```python
from build123d import *

# Parameters (mm, degrees)
ESTRUSIONE_ESTRUSIONE1_DEPTH                 = 5
FORO_LAMATO_PER_VITE_M4_A_TESTA_CILI_2_COUNT = 2
FORO_LAMATO_PER_VITE_M4_A_TESTA_CILI_2_PITCH = 164
FORO_LAMATO_PER_VITE_M4_A_TESTA_CILI_3_COUNT = 2
FORO_LAMATO_PER_VITE_M4_A_TESTA_CILI_3_PITCH = 159
SCHIZZO5_R                                   = 1.75
SCHIZZO5_R_2                                 = 10
SCHIZZO5_R_3                                 = 11
SCHIZZO5_R_4                                 = 13
SCHIZZO5_R_5                                 = 4
SCHIZZO5_R_6                                 = 26
SCHIZZO5_W                                   = 39
SCHIZZO5_H                                   = 24
TAGLIO_ESTRUSIONE2_DEPTH                     = 7


with BuildPart() as part:
    # Schizzo1 → Estrusione-Estrusione1 (new body)
    with BuildSketch(Plane.XY):
        with BuildLine():
            Line((0, 20), (0, 168))
            ThreePointArc((0, 168), (5.857864376, 182.142135624), (20, 188))
            Line((20, 188), (163, 188))
            ThreePointArc((163, 188), (177.142135624, 182.142135624), (183, 168))
            Line((183, 168), (183, 150.284271247))
            ThreePointArc((183, 150.284271247), (181.47759065, 142.6306026), (177.142135624, 136.142135624))
            Line((177.142135624, 136.142135624), (46.857864376, 5.857864376))
            ThreePointArc((46.857864376, 5.857864376), (40.3693974, 1.52240935), (32.715728753, 0))
            Line((32.715728753, 0), (20, 0))
            ThreePointArc((20, 0), (5.857864376, 5.857864376), (0, 20))
        make_face()
    extrude(amount=ESTRUSIONE_ESTRUSIONE1_DEPTH)

    # Schizzo4 → Foro lamato per Vite M4 a testa cilindrica piana-1 (revolve, cut)
    with BuildSketch(Plane(origin=(12, 176, 5), x_dir=(0, -1, 0), z_dir=(1, 0, 0))):
        Polygon((0, 0), (0, 5), (2.25, 5), (2.25, 2.6), (4, 2.6), (4, 0.025), (4.025, 0), align=None)
    foro_lamato_per_vite_m4_a_testa_cilindri = revolve(axis=Axis((12, 176, 11.35), (0, 0, -1)), mode=Mode.SUBTRACT)

    # Foro lamato per Vite M4 a testa cili 2: Foro lamato per Vite M4 a testa cilindrica piana-1 ×2
    with Locations(*[(0, -i * FORO_LAMATO_PER_VITE_M4_A_TESTA_CILI_2_PITCH, 0) for i in range(1, FORO_LAMATO_PER_VITE_M4_A_TESTA_CILI_2_COUNT)]):
        add(foro_lamato_per_vite_m4_a_testa_cilindri, mode=Mode.SUBTRACT)

    # Foro lamato per Vite M4 a testa cili 3: Foro lamato per Vite M4 a testa cilindrica piana-1 ×2
    with Locations(*[(i * FORO_LAMATO_PER_VITE_M4_A_TESTA_CILI_3_PITCH, 0, 0) for i in range(1, FORO_LAMATO_PER_VITE_M4_A_TESTA_CILI_3_COUNT)]):
        add(foro_lamato_per_vite_m4_a_testa_cilindri, mode=Mode.SUBTRACT)

    # Schizzo5 → Taglio-Estrusione2 (cut)
    with BuildSketch(Plane.XY.offset(5)):
        with Locations((12, 32)):
            Circle(SCHIZZO5_R)
        with Locations((58.5, 32)):
            Circle(SCHIZZO5_R)
        with Locations((20, 70)):
            Circle(SCHIZZO5_R_2)
        with Locations((20, 138)):
            Circle(SCHIZZO5_R_3)
        with Locations((30, 105)):
            Circle(SCHIZZO5_R_4)
        with Locations((40, 178)):
            Circle(SCHIZZO5_R_5)
        with Locations((78, 178)):
            Circle(SCHIZZO5_R_5)
        with Locations((116, 178)):
            Circle(SCHIZZO5_R_5)
        with Locations((154, 178)):
            Circle(SCHIZZO5_R_5)
        with Locations((68, 138)):
            Circle(SCHIZZO5_R_6)
        with Locations((133, 138)):
            Circle(SCHIZZO5_R_6)
        with Locations((68, 73)):
            Circle(SCHIZZO5_R_6)
        with Locations((35.25, 32)):
            Rectangle(SCHIZZO5_W, SCHIZZO5_H)
    extrude(amount=-TAGLIO_ESTRUSIONE2_DEPTH, mode=Mode.SUBTRACT)


solid = part.part
```
Design review of the part built by this model. Coordinates are the model's own, in mm. A direction names the side the tool comes from. Give positions to 0.01 mm unless a question says otherwise; leave off trailing zeros. Write each loop counter-clockwise with the first axis right and the second up, starting at its lowest first coordinate (ties: lowest second). Pieces come first, ordered by that corner, then holes. Notation, with made-up numbers: (71.5, 36) - (97.5, 36) arc R20 cw to (97.5, 75) - close; hole circle Ø3 at (3.5, 86.5). An arc over 180 degrees is marked (long way). Return JSON: item names as keys, results as strings. Group by question number.
(1) We need section D-D, the plane x = 125.5. Give the boundary of the cut face in (y, z), then the cut area to 3 significant figures.
(2) Mouldability with a two-part tool opening along Y and no side actions: class faces 1 (the flat face through (93, 116, 0)), 2 (the cylindrical face through (181.52, 142.73, 2.46)), 3 (the cylindrical face through (167.627, 173.85, 3.706)), 4 (the cylindrical face through (5.703, 181.986, 2.465)) as +Y half, -Y half, draft (parallel to the pull), parting line (faces both ways), or undercut.
(3) We need section B-B, the plane z = 1.1. Give the number of separate pieces and of enclosed holes in the cut face, then the cut area to 3 significant figures.
(4) We need section A-A, the plane x = 78. Give the boundary of the cut face in (y, z).
(5) Insertion check: pin 1 (5.5 mm diameter, centred on x = 58.5, y = 32, fed in from -Z); pin 2 (1 mm diameter, centred on y = 102.5, z = 2, fed in from +X); pin 3 (17.5 mm diameter, centred on x = 20, y = 138, fed in from +Z); pin 4 (2 mm diameter, centred on x = 61.5, z = 2.5, fed in from -Y). Each pin has a flat end and moves straight along its axis. Give the tip position at first contact, or say it passes through.
(6) To check wall thickness, follow probe 1 along X at (y, z) = (77, 2.7); probe 2 along Y at (x, z) = (12, 3.2); probe 3 along Y at (x, z) = (20, 3.5). State the ranges of each line that lie inside material, in increasing order.
(7) We need section C-C, the plane y = 40. Give the boundary of the cut face in (x, z).
(8) Machinability: for faces 5 (the cylindrical face through (6.014, 5.703, 2.465)), 6 (the flat face through (14, 178, 2.4)), 7 (the flat face through (54.75, 32, 3)), which of the approach directions +Z, -Z, +X, -X, +Y, -Y give a long, thin tool a straight path to every point of the face, cutting with its end or side? Answer none if there is none.
Reported:
{
 "1": {"outline": "(84.5, 0) - (113.11, 0) - (113.11, 5) - (84.5, 5) - close; (162.89, 0) - (188, 0) - (188, 5) - (162.89, 5) - close", "area": "269 mm2"},
 "2": {"face 1": "draft", "face 2": "-Y half", "face 3": "undercut", "face 4": "+Y half"},
 "3": {"separate pieces": "1", "enclosed holes": "16", "area": "15,200 mm2"},
 "4": {"outline": "(37, 0) - (49, 0) - (49, 5) - (37, 5) - close; (97, 0) - (114, 0) - (114, 5) - (97, 5) - close; (162, 0) - (174, 0) - (174, 5) - (162, 5) - close; (182, 0) - (188, 0) - (188, 5) - (182, 5) - close"},
 "5": {"pin 1": "stops at z = 0", "pin 2": "stops at x = 144", "pin 3": "passes through", "pin 4": "stops at y = 19.5"},
 "6": {"probe 1": "x = 0 to 12.86, 27.14 to 42.31, 93.69 to 118", "probe 2": "y = 1.67 to 8, 16 to 30.25, 33.75 to 64, 76 to 130.45, 145.55 to 172, 180 to 186.33", "probe 3": "y = 0 to 20, 44 to 60, 80 to 96.69, 113.31 to 127, 149 to 188"},
 "7": {"outline": "(0, 0) - (15.75, 0) - (15.75, 5) - (0, 5) - close; (54.75, 0) - (81, 0) - (81, 5) - (54.75, 5) - close"},
 "8": {"face 5": "+Z, -Z, -X, -Y", "face 6": "+Z", "face 7": "+Z, -Z"}
}
